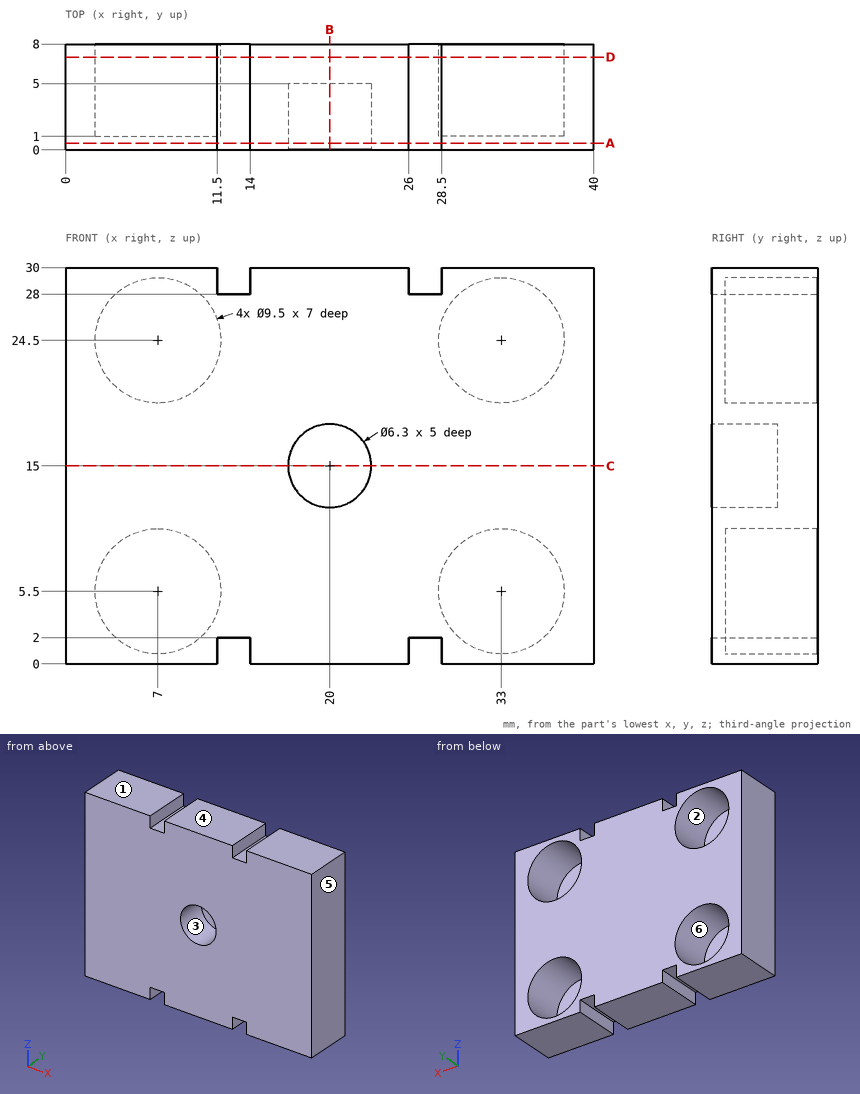
Geometry: see drawing. Coordinates: mm, zero at the bounding-box minimum. A direction names the side the tool comes from. Give positions to 0.01 mm unless a question says otherwise; leave off trailing zeros. Loops run counter-clockwise (first coordinate to the right, second up) from the corner with the lowest first, then second, coordinate; pieces in that order, holes last. Notation, with made-up numbers: (8.25, -19) - (42.25, -19) arc R28 cw to (42.25, 6) - close; hole circle Ø3 at (2.5, 47). An arc over 180 degrees is marked (long way). One line per question, with ' | ' between items. Start each with the question number.
(1) Section query C-C on z = 15. Return loops of the section in (x, y), then the cut area to 4 significant figures.
(2) Ray query, line 1 (X direction, y = 4.75, z = 5.5); line 2 (X direction, y = 1.75, z = 2.75); line 3 (X direction, y = 2.7, z = 15). Return the intervals inside material, ascending. Write a range as from..to.
(3) Section query D-D on y = 7. Return loops of the section in (x, z), then the cut area to 3 significant figures.
(4) Reachability of the marked faces 1, 2 and 3 from +Z, -Z, +X, -X, +Y, -Y: full face, straight path, thin tool, end or side. Return the list, or none.
(5) Pull-direction query (X, two-part tool) for the marked faces 4, 5 and 6; classes: released by +X, released by -X, zero draft, split by the parting line, or undercut.
(6) Section query A-A on y = 0.5. Return loops of the section in (x, z), then the cut area to 3 significant figures.
(7) Contact query for flat-ended pins moving along their axis: pin 1 (1.2 mm diameter, centred on x = 13, y = 5, fed in from -Z); pin 2 (3 mm diameter, centred on x = 7.5, z = 4, fed in from +Y). Output: stop coordinate, or through.
(8) Section query B-B on x = 20. Return loops of the section in (y, z).
The answers:
1) outline: (0, 0) - (16.85, 0) - (16.85, 5) - (23.15, 5) - (23.15, 0) - (40, 0) - (40, 8) - (0, 8) - close | area: 288.5 mm2
2) line 1: 0..2.25, 11.75..28.25, 37.75..40 | line 2: 0..3.13, 10.87..29.13, 36.87..40 | line 3: 0..16.85, 23.15..40
3) outline: (0, 0) - (11.5, 0) - (11.5, 2) - (14, 2) - (14, 0) - (26, 0) - (26, 2) - (28.5, 2) - (28.5, 0) - (40, 0) - (40, 30) - (28.5, 30) - (28.5, 28) - (26, 28) - (26, 30) - (14, 30) - (14, 28) - (11.5, 28) - (11.5, 30) - (0, 30) - close; hole circle Ø9.5 at (7, 5.5); hole circle Ø9.5 at (7, 24.5); hole circle Ø9.5 at (33, 5.5); hole circle Ø9.5 at (33, 24.5) | area: 896 mm2
4) face 1: +Z, +X, -X, +Y, -Y | face 2: +Y | face 3: -Y
5) face 4: zero draft | face 5: released by +X | face 6: undercut
6) outline: (0, 0) - (11.5, 0) - (11.5, 2) - (14, 2) - (14, 0) - (26, 0) - (26, 2) - (28.5, 2) - (28.5, 0) - (40, 0) - (40, 30) - (28.5, 30) - (28.5, 28) - (26, 28) - (26, 30) - (14, 30) - (14, 28) - (11.5, 28) - (11.5, 30) - (0, 30) - close; hole circle Ø6.3 at (20, 15) | area: 1,150 mm2
7) pin 1: z = 2 | pin 2: y = 1
8) outline: (0, 0) - (8, 0) - (8, 30) - (0, 30) - (0, 18.15) - (5, 18.15) - (5, 11.85) - (0, 11.85) - close
